```python
from build123d import *

# Parameters (mm, degrees)
F1_DEPTH = 720
F2_DEPTH = 25
F3_R     = 5


with BuildPart() as f1:
    # F0 (on Top) → F1 (new body)
    with BuildSketch(Plane.XY):
        Polygon((451.088522, 564.315002), (-448.911478, 564.315002), (-448.911478, -335.684998), (111.088522, -335.684998), (111.088522, 4.315002), (451.088522, 4.315002), align=None)
        Polygon((-430.911478, -317.684998), (-430.911478, 546.315002), (433.088522, 546.315002), (433.088522, 22.315002), (93.088522, 22.315002), (93.088522, -317.684998), align=None, mode=Mode.SUBTRACT)
    extrude(amount=F1_DEPTH)

    # F0 (on Top) → F2 (join)
    with BuildSketch(Plane.XY):
        Polygon((433.088522, 546.315002), (-430.911478, 546.315002), (-430.911478, -317.684998), (93.088522, -317.684998), (93.088522, 22.315002), (433.088522, 22.315002), align=None)
    extrude(amount=F2_DEPTH)

    # F3
    f3_edges = [f1.edges().sort_by_distance(p)[0] for p in [
        (451.088522, 4.315002, 360),
        (111.088522, 4.315002, 360),
        (111.088522, -335.684998, 360),
        (281.088522, 4.315002, 720),
        (111.088522, -165.684998, 720),
    ]]
    fillet(f3_edges, radius=F3_R)


solid = f1.part
```
Verification items for the finished model (mm, model axes). A direction names the side the tool comes from. Give positions to 0.01 mm unless a question says otherwise; leave off trailing zeros. Order: outer loops, then holes, each group sorted by start corner. A loop starts at its lowest first (then second) coordinate and runs counter-clockwise, first axis right, second up. Notation, with made-up numbers: (13.25, 11) - (51.25, 11) arc R12 ccw to (51.25, 33) - close; hole circle Ø7 at (32, -10). An arc over 180 degrees is marked (long way). Answer as CSV lines item,"result". Start each with the question number.
Item 1: Gauge pin test, flat ends, axial feed: pin 1 (8 mm diameter, centred on x = 191.5, y = 19.5, fed in from -Z); pin 2 (4 mm diameter, centred on x = 133, z = 451.5, fed in from -Y) (3 decimals). Record the tip position at first contact, or that the pin passes through.
Item 2: Access from +Z, -Z, +X, -X, +Y, -Y to the whole of each face (thin tool, end or side, straight path). Record for faces 4 (the face through (-175, -335.685, 355)), 5 (the face through (-5, 120, 25)), 6 (the face through (111.089, -168, 352)).
Item 3: Material ranges on L1, parallel to Y at x = 84, z = 323.5 (3 decimals); L2, parallel to Y at x = 175.5, z = 379.5 (3 decimals); L3, parallel to X at y = 332, z = 406, recorded low to high.
Item 4: Mould release check, pull along X, two halves, no side actions. Record for faces 1 (the face through (7, 564.315, 355)), 2 (the face through (265, 22.315, 368)), 3 (the face through (451.089, 283, 355)): released by +X, released by -X, zero draft, split by the parting line, or undercut.
Item 5: Section check A-A, the plane z = 157.5. Record the boundary of the cut face in (x, y) (3 decimals).
Item 6: Section check B-B, the plane y = 333. Record the boundary of the cut face in (x, z), plus the area to 3 significant figures.
Item 7: Section check C-C, the plane x = -197. Record the boundary of the cut face in (y, z) (3 decimals).
Item 8: Section check D-D, the plane y = -91. Record the boundary of the cut face in (x, z), plus the area to 3 significant figures.
Filled in:
1,pin 1,"z = 0"
1,pin 2,"y = 4.315"
2,face 4,"+Z, -Z, +X, -X, -Y"
2,face 5,"+Z"
2,face 6,"+Z, -Z, +X, -Y"
3,L1,"-335.685 to -317.685, 546.315 to 564.315"
3,L2,"4.315 to 22.315, 546.315 to 564.315"
3,L3,"-448.91 to -430.91, 433.09 to 451.09"
4,face 1,"zero draft"
4,face 2,"undercut"
4,face 3,"released by +X"
5,outline,"(-448.911, -335.685) - (106.089, -335.685) arc R5 ccw to (111.089, -330.685) - (111.089, -0.685) arc R5 cw to (116.089, 4.315) - (446.089, 4.315) arc R5 ccw to (451.089, 9.315) - (451.089, 564.315) - (-448.911, 564.315) - close; hole (-430.911, -317.685) - (93.089, -317.685) - (93.089, 22.315) - (433.089, 22.315) - (433.089, 546.315) - (-430.911, 546.315) - close"
6,outline,"(-448.91, 0) - (451.09, 0) - (451.09, 720) - (433.09, 720) - (433.09, 25) - (-430.91, 25) - (-430.91, 720) - (-448.91, 720) - close"
6,area,"47,500 mm^2"
7,outline,"(-335.685, 0) - (564.315, 0) - (564.315, 720) - (546.315, 720) - (546.315, 25) - (-317.685, 25) - (-317.685, 720) - (-335.685, 720) - close"
8,outline,"(-448.91, 0) - (111.09, 0) - (111.09, 715) arc R5 ccw to (106.09, 720) - (93.09, 720) - (93.09, 25) - (-430.91, 25) - (-430.91, 720) - (-448.91, 720) - close"
8,area,"39,000 mm^2"
